Could you check a few things on this model? Use its own coordinates, in mm. A direction names the side the tool comes from. Give positions to 0.01 mm unless a question says otherwise; leave off trailing zeros. Use CSV: the item, a comma, the result in double quotes.
```python
from build123d import *

# Parameters (mm, degrees)
F0_W     = 100
F0_H     = 25
F1_DEPTH = 3
F2_W     = 2
F2_H     = 21.208797
F3_DEPTH = 25


with BuildPart() as f1:
    # F0 (on Top) → F1 (new body)
    with BuildSketch(Plane.XY):
        with Locations((8.08065, 35.752659)):
            Rectangle(F0_W, F0_H)
    extrude(amount=F1_DEPTH)

    # F2 (on face) → F3 (cut)
    with BuildSketch(Plane.XY.offset(3)):
        with Locations((-24.790619, 28.26475)):
            Rectangle(F2_W, F2_H)
        with Locations((-20.790619, 28.26475)):
            Rectangle(F2_W, F2_H)
        with Locations((-16.790619, 28.26475)):
            Rectangle(F2_W, F2_H)
        with Locations((-12.790619, 28.26475)):
            Rectangle(F2_W, F2_H)
        with Locations((-8.790619, 28.26475)):
            Rectangle(F2_W, F2_H)
        with Locations((-4.790619, 28.26475)):
            Rectangle(F2_W, F2_H)
        with Locations((-0.790619, 28.26475)):
            Rectangle(F2_W, F2_H)
        with Locations((3.209381, 28.26475)):
            Rectangle(F2_W, F2_H)
        with Locations((7.209381, 28.26475)):
            Rectangle(F2_W, F2_H)
        with Locations((11.209381, 28.26475)):
            Rectangle(F2_W, F2_H)
        with Locations((15.209381, 28.26475)):
            Rectangle(F2_W, F2_H)
        with Locations((19.209381, 28.26475)):
            Rectangle(F2_W, F2_H)
        with Locations((23.209381, 28.26475)):
            Rectangle(F2_W, F2_H)
        with Locations((27.209381, 28.26475)):
            Rectangle(F2_W, F2_H)
        with Locations((31.209381, 28.26475)):
            Rectangle(F2_W, F2_H)
        with Locations((35.209381, 28.26475)):
            Rectangle(F2_W, F2_H)
        with Locations((39.209381, 28.26475)):
            Rectangle(F2_W, F2_H)
        with Locations((43.209381, 28.26475)):
            Rectangle(F2_W, F2_H)
        with Locations((47.209381, 28.26475)):
            Rectangle(F2_W, F2_H)
        with Locations((51.209381, 28.26475)):
            Rectangle(F2_W, F2_H)
        with Locations((55.209381, 28.26475)):
            Rectangle(F2_W, F2_H)
    extrude(amount=-F3_DEPTH, mode=Mode.SUBTRACT)


solid = f1.part
```
1. Please list where this line runs through material, in increasing order: line 1 (Y direction, x = -13, z = 2.3).
Outcome:
line 1,"38.87 to 48.25"
2. Which directions (+Z, -Z, +X, -X, +Y, -Y) give clear straight access to the entire face, cutting with the end or side of a thin tool? Please do faces 1 (the face through (7, 41, 3)), 2 (the face through (-17.791, 31, 2)).
Outcome:
face 1,"+Z, +X, -X, +Y, -Y"
face 2,"+Z, -Z, -Y"
3. If we mould it in two halves opening along X, with no side actions, what happens to faces 3 (the face through (-41.919, 36, 1)), 4 (the face through (53, 23.253, 1)), 5 (the face through (4.209, 31, 2))? For each: +X half, -X half, draft (parallel to the pull), parting line (faces both ways), or undercut.
Outcome:
face 3,"-X half"
face 4,"draft"
face 5,"undercut"
4. I want a section at A-A, the plane y = 35.25. Give the number of separate pieces and of enclosed holes in the cut face, then the cut area to 3 significant figures.
Outcome:
separate pieces,"22"
enclosed holes,"0"
area,"174 mm2"
5. I'm going to push a flat-ended pin straight in: pin 1 Ø0.6 at (x, z) = (43.5, 2) entering from -Y. Where does the tip first touch, or does it pass through?
Outcome:
pin 1,"y = 38.87"
